Model file for the job. Use its own axes, mm. Face numbers are marked on the shaded views. A direction names the side the tool comes from. Round coordinates to 2 decimals unless told otherwise and drop trailing zeros. Order: outer loops, then holes, each group sorted by start corner. A loop starts at its lowest first (then second) coordinate and runs counter-clockwise, first axis right, second up. Notation, with made-up numbers: M -1.75,-32 L 43.25,-32 A8 ccw 43.25,-25 Z; hole C -16,-39 d11. An arc over 180 degrees is marked long. Return JSON: item names as keys, results as strings. Group by question number.
Item 1: Slice it at C-C on y = 30. Write the cut outline in (x, z).
Item 2: Pin check, flat tips, straight feed: pin 1 Ø12 at (x, z) = (25, 20) entering from -Y; pin 2 Ø1 at (x, y) = (27.5, -1) entering from -Z; pin 3 Ø0.6 at (x, y) = (34, -1) entering from +Z; pin 4 Ø1 at (x, z) = (6.5, 26) entering from +Y. Stop position of each tip, or through.
Item 3: Slice it at B-B on z = 15. Write the cut outline in (x, y).
Item 4: Slice it at A-A on x = 31. Write the cut outline in (y, z), then the cut area to 3 significant figures.
Item 5: Which spindle directions (+Z, -Z, +X, -X, +Y, -Y) get a long thin tool onto all of the face, cutting with end or side? Do the marked faces 1 and 2. Say none if no direction does.
Item 6: Slice it at D-D on z = 20. Write the cut outline in (x, y), then the cut area to 3 significant figures.
Item 7: Probe line 1 along Y through (x, z) = (-0.8, 20); line 2 along Z through (x, y) = (25, -1.1); line 3 along X through (y, z) = (1, 3.5). List the from-to ranges inside material, lowest first.
from build123d import *

# Parameters (mm, degrees)
RESSALTO_EXTRUS_O1_DEPTH = 40
ESBO_O2_R                = 10
CORTE_EXTRUS_O1_DEPTH    = 40
ESBO_O3_R                = 7.5
CORTE_EXTRUS_O2_DEPTH    = 40
FILETE1_R                = 10
ESBO_O4_W                = 50
ESBO_O4_H                = 7.5
CORTE_EXTRUS_O3_DEPTH    = 290


with BuildPart() as part:
    # Esboço1 → Ressalto-extrusão1 (new body)
    with BuildSketch(Plane.XY):
        Polygon((0, 0), (0, 50), (-2, 50), (-2, -2), (50, -2), (50, 0), align=None)
    extrude(amount=RESSALTO_EXTRUS_O1_DEPTH)

    # Esboço2 → Corte-extrusão1 (cut)
    with BuildSketch(Plane(origin=(0, 0, 0), x_dir=(0, 0, -1), z_dir=(1, 0, 0))):
        with Locations((-20, 30)):
            Circle(ESBO_O2_R)
    extrude(amount=-CORTE_EXTRUS_O1_DEPTH, mode=Mode.SUBTRACT)

    # Esboço3 → Corte-extrusão2 (cut)
    with BuildSketch(Plane(origin=(0, 0, 0), x_dir=(1, 0, 0), z_dir=(0, 1, 0))):
        with Locations(Location((25, -20, 0), (0, 0, 180))):
            Circle(ESBO_O3_R)
    extrude(amount=-CORTE_EXTRUS_O2_DEPTH, mode=Mode.SUBTRACT)

    # Filete1
    filete1_edges = [part.edges().sort_by_distance(p)[0] for p in [
        (-1, 50, 40),
        (-1, 50, 0),
    ]]
    fillet(filete1_edges, radius=FILETE1_R)

    # Esboço4 → Corte-extrusão3 (cut)
    with BuildSketch(Plane(origin=(0, 0, 0), x_dir=(1, 0, 0), z_dir=(0, 1, 0))):
        with Locations((25, -36.25)):
            Rectangle(ESBO_O4_W, ESBO_O4_H)
        with Locations((25, -3.75)):
            Rectangle(ESBO_O4_W, ESBO_O4_H)
    extrude(amount=-CORTE_EXTRUS_O3_DEPTH, mode=Mode.SUBTRACT)


solid = part.part
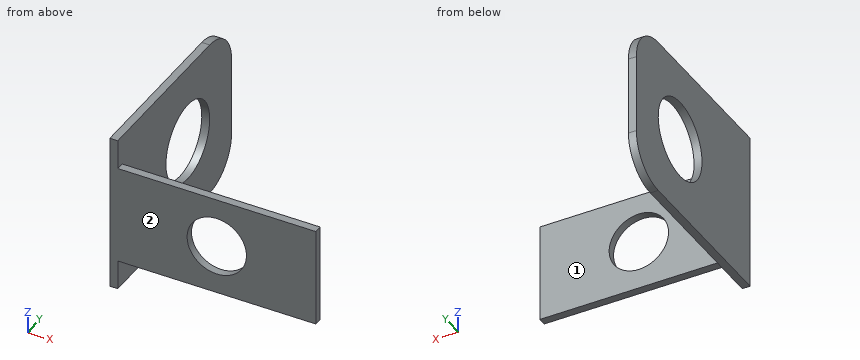
Output values:
{
 "1": {"outline": "M -2,0 L 0,0 L 0,10 L -2,10 Z; M -2,30 L 0,30 L 0,40 L -2,40 Z"},
 "2": {"pin 1": "through", "pin 2": "z = 7.5", "pin 3": "z = 32.5", "pin 4": "y = 0"},
 "3": {"outline": "M -2,-2 L 19.41,-2 L 19.41,0 L 0,0 L 0,21.34 L -2,21.34 Z; M -2,38.66 L 0,38.66 L 0,50 L -2,50 Z; M 30.59,-2 L 50,-2 L 50,0 L 30.59,0 Z"},
 "4": {"outline": "M -2,7.5 L 0,7.5 L 0,15.5 L -2,15.5 Z; M -2,24.5 L 0,24.5 L 0,32.5 L -2,32.5 Z", "area": "32.0 mm²"},
 "5": {"face 1": "+Z, -Z, +X, +Y", "face 2": "+Z, -Z, +X, -X, -Y"},
 "6": {"outline": "M -2,-2 L 17.5,-2 L 17.5,0 L 0,0 L 0,20 L -2,20 Z; M -2,40 L 0,40 L 0,50 L -2,50 Z; M 32.5,-2 L 50,-2 L 50,0 L 32.5,0 Z", "area": "134 mm²"},
 "7": {"line 1": "-2 to 20, 40 to 50", "line 2": "7.5 to 12.5, 27.5 to 32.5", "line 3": "-2 to 0"}
}
